```python
from build123d import *

# Parameters (mm, degrees)
F0_W     = 18
F0_H     = 14
F3_DEPTH = 3
F1_W     = 12.000005
F1_H     = 2.5
F4_DEPTH = 25
F2_W     = 11.083636
F2_H     = 3.694546
F5_DEPTH = 4
F6_R     = 1


with BuildPart() as f3:
    # F0 (on Top) → F3 (new body)
    with BuildSketch(Plane.XY):
        with Locations((9, -7)):
            Rectangle(F0_W, F0_H)
    extrude(amount=F3_DEPTH)

    # F1 (on face) → F4 (cut)
    with BuildSketch(Plane.XY):
        with Locations((9.000003, -4.25)):
            Rectangle(F1_W, F1_H)
        with Locations((9.000003, -9.742595)):
            Rectangle(F1_W, F1_H)
    extrude(amount=F4_DEPTH, mode=Mode.SUBTRACT)

    # F2 (on face) → F5 (join)
    with BuildSketch(Plane.XY):
        with Locations((8.988467, -7.016157)):
            Rectangle(F2_W, F2_H)
    extrude(amount=F5_DEPTH)

    # F6
    f6_edges = [f3.edges().sort_by_distance(p)[0] for p in [
        (8.988467, -8.86343, 4),
        (8.988467, -5.168884, 4),
        (9.000002, -3, 3),
        (9.000002, -10.992595, 3),
        (9, -14, 3),
        (9, 0, 3),
    ]]
    fillet(f6_edges, radius=F6_R)


solid = f3.part
```
Source: CAD feature listing. Evaluate the final solid. Frame: model axes, mm. A direction names the side the tool comes from. Round coordinates to 2 decimals unless told otherwise and drop trailing zeros. Loops run counter-clockwise (first coordinate to the right, second up) from the corner with the lowest first, then second, coordinate; pieces in that order, holes last.
(1) Pull-direction query (Y, two-part tool) for faces 1 (the flat face through (3, -4, 1)), 2 (the flat face through (18, -7, 1)), 3 (the cylindrical face through (9.066, -5.454, 3.699)), 4 (the cylindrical face through (9.126, -13.699, 2.715)); classes: +Y half, -Y half, draft (parallel to the pull), parting line (faces both ways), or undercut.
From the geometry:
face 1: undercut
face 2: draft
face 3: +Y half
face 4: -Y half
(2) Section query D-D (y = -7.5). Output: boundary loops of the cut face in (x, z), and give its area (3 significant figures).
From the geometry:
outline: (0, 0) - (18, 0) - (18, 3) - (14.53, 3) - (14.53, 4) - (3.45, 4) - (3.45, 3) - (0, 3) - close
area: 65.1 mm2
(3) Material intervals for probe 1 along Y at (x, z) = (12.75, 1.7); probe 2 along Z at (x, y) = (17.25, -12.75); probe 3 along X at (y, z) = (-10.75, 0.55), sorted ascending.
From the geometry:
probe 1: y = -14 to -10.99, -8.86 to -5.17, -3 to 0
probe 2: z = 0 to 3
probe 3: x = 0 to 3, 15 to 18
(4) Section query A-A (y = -3.5). Output: boundary loops of the cut face in (x, z).
From the geometry:
outline: (0, 0) - (3, 0) - (3, 3) - (0, 3) - close; (15, 0) - (18, 0) - (18, 3) - (15, 3) - close
(5) Access query for faces 5 (the flat face through (9, -3, 1)), 6 (the cylindrical face through (9.126, -0.301, 2.715)), 7 (the flat face through (14.53, -7, 3.3)). Directions: +Z, -Z, +X, -X, +Y, -Y. A direction counts if a zero-diameter tool reaches every point of the face in a straight line with its end or side. Return the directions, or none.
From the geometry:
face 5: +Z, -Z
face 6: +Z, +X, -X, +Y
face 7: +Z
(6) Section query B-B (x = 5.5). Output: boundary loops of the cut face in (y, z).
From the geometry:
outline: (-14, 0) - (-10.99, 0) - (-10.99, 2) arc R1 ccw to (-11.99, 3) - (-13, 3) arc R1 ccw to (-14, 2) - close; (-8.86, 0) - (-5.17, 0) - (-5.17, 3) arc R1 ccw to (-6.17, 4) - (-7.86, 4) arc R1 ccw to (-8.86, 3) - close; (-3, 0) - (0, 0) - (0, 2) arc R1 ccw to (-1, 3) - (-2, 3) arc R1 ccw to (-3, 2) - close
(7) Contact query for a flat-ended pin moving along its axis: pin 1 Ø6 at (x, y) = (8, -1.5) entering from -Z. Output: stop coordinate, or through.
From the geometry:
pin 1: stops at z = 0
(8) Section query C-C (z = 0.95). Output: boundary loops of the cut face in (x, y).
From the geometry:
outline: (0, -14) - (18, -14) - (18, 0) - (0, 0) - close; hole (3, -10.99) - (15, -10.99) - (15, -8.49) - (14.53, -8.49) - (14.53, -8.86) - (3.45, -8.86) - (3.45, -8.49) - (3, -8.49) - close; hole (3, -5.5) - (3.45, -5.5) - (3.45, -5.17) - (14.53, -5.17) - (14.53, -5.5) - (15, -5.5) - (15, -3) - (3, -3) - close
